```python
from build123d import *

# Parameters (mm, degrees)
F1_DEPTH = 17.78
F2_R     = 3.175
F3_DEPTH = 2.541


with BuildPart() as f1:
    # F0 (on Top) → F1 (new body)
    with BuildSketch(Plane.XY):
        with BuildLine():
            Line((-16.804146, -14.937672), (-29.504146, -14.937672))
            Line((-29.504146, -14.937672), (-29.504146, -17.477672))
            Line((-29.504146, -17.477672), (-16.804146, -17.477672))
            Line((-16.804146, -17.477672), (-16.804146, -25.605672))
            ThreePointArc((-16.804146, -25.605672), (-3.596146, -38.813672), (9.611854, -25.605672))
            Line((9.611854, -25.605672), (9.611854, -17.477672))
            Line((9.611854, -17.477672), (22.311854, -17.477672))
            Line((22.311854, -17.477672), (22.311854, -14.937672))
            Line((22.311854, -14.937672), (9.611854, -14.937672))
            Line((9.611854, -14.937672), (7.071854, -14.937672))
            Line((7.071854, -14.937672), (7.071854, -25.605672))
            ThreePointArc((7.071854, -25.605672), (-3.596146, -36.273672), (-14.264146, -25.605672))
            Line((-14.264146, -25.605672), (-14.264146, -14.937672))
            Line((-14.264146, -14.937672), (-16.804146, -14.937672))
        make_face()
    extrude(amount=F1_DEPTH)

    # F2 (on face) → F3 (cut, through all)
    with BuildSketch(Plane.XZ.offset(17.477672)):
        with Locations((-23.154146, 8.89)):
            Circle(F2_R)
        with Locations((15.961854, 8.89)):
            Circle(F2_R)
    extrude(amount=-F3_DEPTH, mode=Mode.SUBTRACT)


solid = f1.part
```
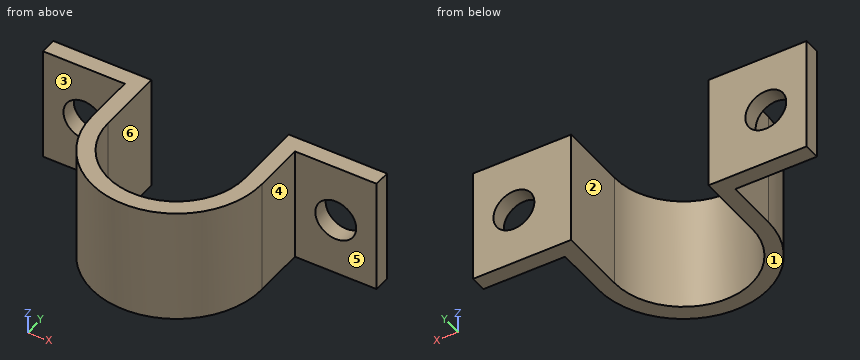
Geometry check sheet. Reference: the model listing, model coordinates, mm. Face numbers are marked on the shaded views. A direction names the side the tool comes from. Coordinates: 2 decimals unless noted, no trailing zeros. Loops run counter-clockwise (first coordinate to the right, second up) from the corner with the lowest first, then second, coordinate; pieces in that order, holes last. Notation, with made-up numbers: (44.25, -25.5) -> (73.25, -25.5) arc R20 ccw to (73.25, -18.5) -> close; hole circle Ø1 at (-1, 52). An arc over 180 degrees is marked (long way). Put each result on its own line as item: value.
1) Thickness scan on line 1 (X direction, y = -24.5, z = 1.75); line 2 (X direction, y = -16, z = 1.25); line 3 (Y direction, x = -19, z = 9.75). Record the ranges inside material, lowest first.
Result set:
line 1: x = -16.8 to -14.26, 7.07 to 9.61
line 2: x = -29.5 to -14.26, 7.07 to 22.31
line 3: y = -17.48 to -14.94
2) Cross-section at D-D on y = -29. Record the boundary of the cut face in (x, z), plus the area to 3 significant figures.
Result set:
outline: (-16.36, 0) -> (-13.71, 0) -> (-13.71, 17.78) -> (-16.36, 17.78) -> close; (6.52, 0) -> (9.17, 0) -> (9.17, 17.78) -> (6.52, 17.78) -> close
area: 94.3 mm^2
3) Gauge pin test, flat ends, axial feed: pin 1 Ø10 at (y, z) = (-26, 8) entering from -X; pin 2 Ø8 at (y, z) = (-33, 6.5) entering from -X; pin 3 Ø8 at (x, y) = (-21.5, -23) entering from -Z; pin 4 Ø4 at (x, z) = (-23, 7.5) entering from -Y. Record the tip position at first contact, or that the pin passes through.
Result set:
pin 1: stops at x = -16.8
pin 2: stops at x = -16.36
pin 3: passes through
pin 4: stops at y = -17.48
4) Cross-section at A-A on y = -23.75. Record the boundary of the cut face in (x, z).
Result set:
outline: (-16.8, 0) -> (-14.26, 0) -> (-14.26, 17.78) -> (-16.8, 17.78) -> close; (7.07, 0) -> (9.61, 0) -> (9.61, 17.78) -> (7.07, 17.78) -> close
5) Release check for a two-part mould opening along X. For the marked faces 4, 5 and 6 record: released by +X, released by -X, zero draft, split by the parting line, or undercut.
Result set:
face 4: released by +X
face 5: zero draft
face 6: undercut
6) Tool access check on the marked faces 1, 2 and 3. Record the directions out of +Z, -Z, +X, -X, +Y, -Y that give a thin tool (end or side, any length) a straight path to the whole face; none if there is none.
Result set:
face 1: -Z, +X, -X, +Y, -Y
face 2: +Z, -Z, +Y
face 3: +Z, -Z, -X, -Y
